Build history of the part. All positions in model axes, mm. A direction names the side the tool comes from. Round coordinates to 2 decimals unless told otherwise and drop trailing zeros. Order: outer loops, then holes, each group sorted by start corner. A loop starts at its lowest first (then second) coordinate and runs counter-clockwise, first axis right, second up. Notation, with made-up numbers: (78.5, -17) -> (123.5, -17) arc R10 ccw to (123.5, -12) -> close; hole circle Ø11 at (14, -1.75). An arc over 180 degrees is marked (long way). Write item = value, one per line.
from build123d import *

# Parameters (mm, degrees)
ESTRUSIONE_ESTRUSIONE1_DEPTH                         = 40
RACCORDO1_R                                          = 1
FORO_LAMATO_PER_BULLONE_M12_A_TESTA_ESAG_D           = 4.5
FORO_LAMATO_PER_BULLONE_M12_A_TESTA_ESAG_DEPTH       = 8.5
FORO_LAMATO_PER_BULLONE_M12_A_TESTA_ESAG_CBORE_D     = 10
FORO_LAMATO_PER_BULLONE_M12_A_TESTA_ESAG_CBORE_DEPTH = 3
FORO_LAMATO_PER_BULLONE_M12_A_TESTA_ESAG_TIP         = 1.351936393
FORO_LAMATO_PER_BULLONE_M12_A_TESTA_2_D              = 4.5
FORO_LAMATO_PER_BULLONE_M12_A_TESTA_2_DEPTH          = 8.5
FORO_LAMATO_PER_BULLONE_M12_A_TESTA_2_CBORE_D        = 10
FORO_LAMATO_PER_BULLONE_M12_A_TESTA_2_CBORE_DEPTH    = 3
FORO_LAMATO_PER_BULLONE_M12_A_TESTA_2_TIP            = 1.351936393
FORO_PER_VITE_M3_1_D                                 = 3.4
FORO_PER_VITE_M3_1_DEPTH                             = 8.5
FORO_PER_VITE_M3_1_TIP                               = 1.021463052


with BuildPart() as part:
    # Schizzo1 → Estrusione-Estrusione1 (new body)
    with BuildSketch(Plane.XY):
        with BuildLine():
            Line((9, 0), (53, 0))
            ThreePointArc((53, 0), (59.363961031, 2.636038969), (62, 9))
            Line((62, 9), (62, 30.52))
            Line((62, 30.52), (60, 37.73))
            Line((60, 37.73), (60, 80))
            Line((60, 80), (56, 80))
            Line((56, 80), (56, 37.73))
            Line((56, 37.73), (58, 30.52))
            Line((58, 30.52), (58, 9))
            ThreePointArc((58, 9), (56.535533906, 5.464466094), (53, 4))
            Line((53, 4), (9, 4))
            ThreePointArc((9, 4), (5.464466094, 5.464466094), (4, 9))
            Line((4, 9), (4, 30.52))
            Line((4, 30.52), (6, 37.73))
            Line((6, 37.73), (6, 80))
            Line((6, 80), (2, 80))
            Line((2, 80), (2, 37.73))
            Line((2, 37.73), (0, 30.52))
            Line((0, 30.52), (0, 9))
            ThreePointArc((0, 9), (2.636038969, 2.636038969), (9, 0))
        make_face()
    extrude(amount=ESTRUSIONE_ESTRUSIONE1_DEPTH)

    # Raccordo1
    raccordo1_edges = [part.edges().sort_by_distance(p)[0] for p in [
        (2, 80, 20),
        (6, 80, 20),
        (56, 80, 20),
        (60, 80, 20),
    ]]
    fillet(raccordo1_edges, radius=RACCORDO1_R)

    # Foro lamato per Bullone M12 a testa esag
    with Locations(Plane.ZY.offset(-2)):
        with Locations((10, 58.5), (30, 58.5)):
            CounterBoreHole(FORO_LAMATO_PER_BULLONE_M12_A_TESTA_ESAG_D / 2, FORO_LAMATO_PER_BULLONE_M12_A_TESTA_ESAG_CBORE_D / 2, FORO_LAMATO_PER_BULLONE_M12_A_TESTA_ESAG_CBORE_DEPTH, depth=FORO_LAMATO_PER_BULLONE_M12_A_TESTA_ESAG_DEPTH)
            with Locations((0, 0, -(FORO_LAMATO_PER_BULLONE_M12_A_TESTA_ESAG_DEPTH + FORO_LAMATO_PER_BULLONE_M12_A_TESTA_ESAG_TIP / 2))):  # 118° drill point
                Cone(0, FORO_LAMATO_PER_BULLONE_M12_A_TESTA_ESAG_D / 2, FORO_LAMATO_PER_BULLONE_M12_A_TESTA_ESAG_TIP, mode=Mode.SUBTRACT)

    # Foro lamato per Bullone M12 a testa  2
    with Locations(Plane(origin=(60, 0, 0), x_dir=(0, 0, -1), z_dir=(1, 0, 0))):
        with Locations((-30, 58.5), (-10, 58.5)):
            CounterBoreHole(FORO_LAMATO_PER_BULLONE_M12_A_TESTA_2_D / 2, FORO_LAMATO_PER_BULLONE_M12_A_TESTA_2_CBORE_D / 2, FORO_LAMATO_PER_BULLONE_M12_A_TESTA_2_CBORE_DEPTH, depth=FORO_LAMATO_PER_BULLONE_M12_A_TESTA_2_DEPTH)
            with Locations((0, 0, -(FORO_LAMATO_PER_BULLONE_M12_A_TESTA_2_DEPTH + FORO_LAMATO_PER_BULLONE_M12_A_TESTA_2_TIP / 2))):  # 118° drill point
                Cone(0, FORO_LAMATO_PER_BULLONE_M12_A_TESTA_2_D / 2, FORO_LAMATO_PER_BULLONE_M12_A_TESTA_2_TIP, mode=Mode.SUBTRACT)

    # Foro per Vite M3-1
    with Locations(Plane(origin=(0, 4, 0), x_dir=(1, 0, 0), z_dir=(0, 1, 0))):
        with Locations((18.5, -20), (43.5, -20)):
            Hole(FORO_PER_VITE_M3_1_D / 2, depth=FORO_PER_VITE_M3_1_DEPTH)
            with Locations((0, 0, -(FORO_PER_VITE_M3_1_DEPTH + FORO_PER_VITE_M3_1_TIP / 2))):  # 118° drill point
                Cone(0, FORO_PER_VITE_M3_1_D / 2, FORO_PER_VITE_M3_1_TIP, mode=Mode.SUBTRACT)


solid = part.part
Q1. Which spindle directions (+Z, -Z, +X, -X, +Y, -Y) get a long thin tool onto all of the face, cutting with end or side? Do faces 1 (the face through (60, 58, 20)), 2 (the face through (5, 57, 12)), 3 (the face through (57, 57, 8)), 4 (the face through (56, 59, 20)), 5 (the face through (6, 5, 20)). Say none if no direction does.
Check values:
face_1 = +Z, -Z, +X, +Y
face_2 = -X
face_3 = +X
face_4 = +Z, -Z, +Y
face_5 = +Z, -Z
Q2. Flat gauge pins, fed straight in: pin 1 (11.5 mm diameter, centred on y = 58.5, z = 10, fed in from +X); pin 2 (1.5 mm diameter, centred on x = 8.5, y = 43.5, fed in from +Z); pin 3 (2 mm diameter, centred on y = 45, z = 7.5, fed in from -X); pin 4 (3 mm diameter, centred on y = 58.5, z = 8, fed in from +X). Where does each tip first touch, or does it go through?
Check values:
pin_1 = 60
pin_2 = through
pin_3 = 2
pin_4 = 57
Q3. Mould opens along Y. For faces 6 (the face through (5, 57, 32)), 7 (the face through (1.014, 34.175, 19.72)), 8 (the face through (5.6, 37.2, 0)) say: released by +Y, released by -Y, zero draft, split by the parting line, or undercut.
Check values:
face_6 = undercut
face_7 = released by +Y
face_8 = zero draft
Q4. Cut at D-D, the plane z = 37.5. List the corners of the cut face in (x, y).
Check values:
outline = (0, 9) arc R9 ccw to (9, 0) -> (53, 0) arc R9 ccw to (62, 9) -> (62, 30.52) -> (60, 37.73) -> (60, 79) arc R1 ccw to (59, 80) -> (57, 80) arc R1 ccw to (56, 79) -> (56, 37.73) -> (58, 30.52) -> (58, 9) arc R5 cw to (53, 4) -> (9, 4) arc R5 cw to (4, 9) -> (4, 30.52) -> (6, 37.73) -> (6, 79) arc R1 ccw to (5, 80) -> (3, 80) arc R1 ccw to (2, 79) -> (2, 37.73) -> (0, 30.52) -> close
Q5. Probe probe 1 along X at (y, z) = (76, 18); probe 2 along Z at (x, y) = (43.5, 1.95); probe 3 along X at (y, z) = (23, 23.5). List the from-to ranges inside material, lowest first.
Check values:
probe_1 = 2 to 6, 56 to 60
probe_2 = 0 to 18.3, 21.7 to 40
probe_3 = 0 to 4, 58 to 62
Q6. Cut at C-C, the plane y = 43. List the corners of the cut face in (x, z).
Check values:
outline = (2, 0) -> (6, 0) -> (6, 40) -> (2, 40) -> close; (56, 0) -> (60, 0) -> (60, 40) -> (56, 40) -> close
Q7. Cut at B-B, the plane x = 18.5. List the corners of the cut face in (y, z), and give its area (3 significant figures).
Check values:
outline = (0, 0) -> (4, 0) -> (4, 18.3) -> (0, 18.3) -> close; (0, 21.7) -> (4, 21.7) -> (4, 40) -> (0, 40) -> close
area = 146 mm²
Q8. Cut at A-A, the plane z = 20. Give the number of separate pieces and of enclosed holes in the cut face, and give its area (3 significant figures).
Check values:
separate_pieces = 3
enclosed_holes = 0
area = 804 mm²
